Model file for the job. Use its own axes, mm. A direction names the side the tool comes from. Give positions to 0.01 mm unless a question says otherwise; leave off trailing zeros. Loops run counter-clockwise (first coordinate to the right, second up) from the corner with the lowest first, then second, coordinate; pieces in that order, holes last. Notation, with made-up numbers: M 31,32.25 L 88,32.25 A25 cw 88,66.25 Z; hole C 48,71.5 d2. An arc over 180 degrees is marked long. Use CSV: the item, a comma, the result in double quotes. Start each with the question number.
(1) Wall check: line 1 along Y through (x, z) = (43, 9.5); line 2 along Y through (x, z) = (10, 17); line 3 along Z through (x, y) = (44.5, -10.5). Give the ranges that are in metal, low to high. Write a range as from..to.
(2) Tool access for faces 4 (the face through (15.407, -4.852, 7.07)), 5 (the face through (8.01, -28.39, 51.04)), 6 (the face through (14.022, -19.781, 0.986)), 7 (the face through (9, -27, 50)): list every direction of +Z, -Z, +X, -X, +Y, -Y with a clear straight run to the whole face (end or side of a thin tool).
(3) Slice it at D-D on x = 11. List the corners of the cut face in (y, z).
(4) Flat gauge pins, fed straight in: P1, Ø1.7, axis at x = 48.52, y = -36, coming from the +Z side; P2, Ø2.5, axis at y = -25.5, z = 44, coming from the +X side; P3, Ø3, axis at y = -20.5, z = 5, coming from the -X side. Where does each tip first touch, or does it go through?
(5) Slice it at A-A on y = -27. State how many separate pieces and enclosed holes the cut face has, and give its area (3 significant figures).
(6) Two-plate mould, pull along Y, no slides. Class faces 1 (the face through (31, 0, 6)), 2 (the face through (10.5, -29.4, 50.3)), 3 (the face through (7, -27, 33)): pulls with the +Y half, pulls with the -Y half, needs draft (parallel to the pull), parting line crosses it, or undercut.
```python
from build123d import *

# Parameters (mm, degrees)
F1_DEPTH  = 40
F2_T      = -2.5
F3_R      = 3.5
F4_DEPTH  = 12
F5_R      = 1.4
F6_DEPTH  = 12.001
F7_W      = 38.9644660941
F7_H      = 40
F8_DEPTH  = 2
F9_SIZE   = 1.99999
F12_DEPTH = 5
F13_R     = 1.75
F14_DEPTH = 12.001
F15_R     = 3
F16_DEPTH = 3
F17_SIZE  = 1.99999


# Not quite as in the source:
# - a fillet or chamfer is up to 0.001 mm smaller than in the source, because OpenCascade refuses the exact size


with BuildPart() as f1:
    # F0 (on Front) → F1 (new body)
    with BuildSketch(Plane.XZ):
        Polygon((12, 12), (0, 0), (52, 0), (52, 12), align=None)
    extrude(amount=F1_DEPTH)

    # F2
    f2_openings = [f1.faces().sort_by_distance(p)[0] for p in [
        (32, -20, 12),
        (26, -20, 0),
    ]]
    offset(amount=F2_T, openings=f2_openings, kind=Kind.INTERSECTION)

    # F3 (on face) → F4 (join, through all)
    with BuildSketch(Plane.XY.offset(12)):
        with Locations((16.517766953, -36)):
            Circle(F3_R)
        with Locations((48.517766953, -36)):
            Circle(F3_R)
        with Locations((48.517766953, -4)):
            Circle(F3_R)
        with Locations((16.517766953, -4)):
            Circle(F3_R)
    extrude(amount=-F4_DEPTH)

    # F5 (on face) → F6 (cut, through all)
    with BuildSketch(Plane.XY.offset(12)):
        with Locations((16.517766953, -4)):
            Circle(F5_R)
        with Locations((48.517766953, -4)):
            Circle(F5_R)
        with Locations((48.517766953, -36)):
            Circle(F5_R)
        with Locations((16.517766953, -36)):
            Circle(F5_R)
    extrude(amount=-F6_DEPTH, mode=Mode.SUBTRACT)

    # F7 (on face) → F8 (join)
    with BuildSketch(Plane(origin=(0, 0, 0), x_dir=(1, 0, 0), z_dir=(0, 0, -1))):
        with Locations((32.517766953, 20)):
            Rectangle(F7_W, F7_H)
    extrude(amount=-F8_DEPTH)

    # F9 (size 2 in the source; OpenCascade refuses exactly that, so slightly less here)
    f9_edges = [f1.edges().sort_by_distance(p)[0] for p in [
        (13.035534, -20, 2),
    ]]
    chamfer(f9_edges, length=F9_SIZE)

    # F11 (on offset) → F12 (join, symmetric)
    with BuildSketch(Plane.XZ.offset(27)):
        Polygon((7, 59), (7, 7), (12, 12), (12, 59), align=None)
    extrude(amount=F12_DEPTH, both=True)

    # F13 (on face) → F14 (cut, through all)
    with BuildSketch(Plane.YZ.offset(12)):
        with Locations((-27, 52.1)):
            Circle(F13_R)
    extrude(amount=-F14_DEPTH, mode=Mode.SUBTRACT)

    # F15 (on face) → F16 (cut)
    with BuildSketch(Plane.YZ.offset(12)):
        with Locations((-27, 52.1)):
            Circle(F15_R)
    extrude(amount=-F16_DEPTH, mode=Mode.SUBTRACT)

    # F17 (size 2 in the source; OpenCascade refuses exactly that, so slightly less here)
    f17_edges = [f1.edges().sort_by_distance(p)[0] for p in [
        (12, -32, 35.5),
    ]]
    chamfer(f17_edges, length=F17_SIZE)


solid = f1.part
```
Reply:
1,line 1,"y = -40..-37.5, -2.5..0"
1,line 2,"y = -32..-22"
1,line 3,"z = 0..2"
2,face 4,"+Z"
2,face 5,"+X, -X"
2,face 6,"none"
2,face 7,"+X"
3,outline,"M -40,0 L -37.5,0 L -37.5,7.46 L -2.5,7.46 L -2.5,0 L 0,0 L 0,11 L -22,11 L -22,59 L -31,59 L -31,11 L -40,11 Z; hole C -27,52.1 d6"
4,P1,"stops at z = 2"
4,P2,"stops at x = 12"
4,P3,"stops at x = 3.5"
5,separate pieces,"3"
5,enclosed holes,"0"
5,area,"366 mm^2"
6,face 1,"pulls with the +Y half"
6,face 2,"undercut"
6,face 3,"needs draft"
